Geometry check sheet. Reference: the model listing, model coordinates, mm. A direction names the side the tool comes from. Coordinates: 2 decimals unless noted, no trailing zeros. Write each loop counter-clockwise with the first axis right and the second up, starting at its lowest first coordinate (ties: lowest second). Pieces come first, ordered by that corner, then holes. Notation, with made-up numbers: (8, 51) -> (21, 51) arc R31 cw to (21, 89) -> close; hole circle Ø1 at (77, 7). An arc over 180 degrees is marked (long way). Use a Markdown table: item, result.
```python
from build123d import *

# Parameters (mm, degrees)
F1_DEPTH      = 6.35
F2_W          = 1.3509193668
F2_H          = 10.8486381359
F3_DEPTH      = 2
F5_DEPTH      = 3
F7_R          = 5
F8_T1_DEPTH   = 22.7018387336
F9_T1_DEPTH   = 22.7018387336
F10_T1_DEPTH  = 37.7293119504
F11_T1_DEPTH  = 50.3092406281
F11_T3_DEPTH  = 50.3092406281
F11_T8_DEPTH  = 71.0975509994
F11_T13_DEPTH = 71.0975509994
F12_R         = 1
F13_R         = 1
F14_R         = 1
F15_R         = 1


# Not quite as in the source:
# - a fillet or chamfer that OpenCascade refuses, or shapes differently, is made with other operations: its cross-section is extruded or revolved along the edge and cut away or added


with BuildPart() as f1:
    # F0 (on Top) → F1 (new body)
    with BuildSketch(Plane.XY):
        Polygon((0, -66.0772249103), (0, 35.7286036015), (-4.0004998446, 10.6220170856), (-4.0004998446, -13.1050860509), (-33.7973274291, -28.5552926362), (-33.7973274291, -40.1429459453), (-4.2763971724, -40.1429459453), (-4.2763971724, -50.6270192564), (-13.1050860509, -62.766470015), (-13.1050860509, -69.3879872561), align=None)
    extrude(amount=F1_DEPTH)

    # F2 (on face) → F3 (join)
    with BuildSketch(Plane.XY.offset(6.35)):
        with Locations((-0.6754596834, 8.3060876932)):
            Rectangle(F2_W, F2_H)
    extrude(amount=F3_DEPTH)

    # F4 (on Right) → F5 (join)
    with BuildSketch(Plane.YZ):
        with BuildLine():
            Line((-69.653019309, 0), (-54.4461198151, 0))
            Line((-54.4461198151, 0), (-59.1908343158, 12.4009543867))
            ThreePointArc((-59.1908343158, 12.4009543867), (-61.0264090525, 14.733305135), (-63.8606947699, 15.6142245978))
            Line((-63.8606947699, 15.6142245978), (-66.3944035769, 15.6142245978))
            Line((-66.3944035769, 15.6142245978), (-69.653019309, 0))
        make_face()
    extrude(amount=-F5_DEPTH)

    # F6: F1 across face


with BuildPart() as f1_1:
    add(f1.part)
    add(f1.part.mirror(Plane(origin=(0, -20.6881401181, 4.0270783), x_dir=(0, 1, 0), z_dir=(1, 0, 0))))

    # F7
    f7_edges = [f1_1.edges().sort_by_distance(p)[0] for p in [
        (-18.898914, -20.830189, 6.35),
        (18.898914, -20.830189, 6.35),
    ]]
    fillet(f7_edges, radius=F7_R)

    # F8: fillet of radius 5 on 1 edges, made by hand

    # F8_s2 → F8_t1 (cut)
    with BuildSketch(Plane.YZ.offset(-11.3509193668)):
        with BuildLine():
            ThreePointArc((13.7304067612, 6.35), (11.9664747387, 7.822135955), (9.7304067612, 8.35))
            Line((9.7304067612, 8.35), (13.7304067612, 8.35))
            Line((13.7304067612, 8.35), (13.7304067612, 6.35))
        make_face()
    extrude(amount=F8_T1_DEPTH, mode=Mode.SUBTRACT)

    # F9: fillet of radius 5 on 1 edges, made by hand

    # F9_s2 → F9_t1 (cut)
    with BuildSketch(Plane.YZ.offset(-11.3509193668)):
        with BuildLine():
            ThreePointArc((2.8817686252, 6.35), (4.6457006477, 7.822135955), (6.8817686252, 8.35))
            Line((6.8817686252, 8.35), (2.8817686252, 8.35))
            Line((2.8817686252, 8.35), (2.8817686252, 6.35))
        make_face()
    extrude(amount=F9_T1_DEPTH, mode=Mode.SUBTRACT)

    # F10: fillet of radius 1 on 1 edges, made by hand

    # F10_s2 → F10_t1 (cut)
    with BuildSketch(Plane.XY.offset(-15.6896559752)):
        with BuildLine():
            ThreePointArc((-0.9875420089, 29.5309258493), (0, 30.3735702625), (0.9875420089, 29.5309258493))
            Line((0.9875420089, 29.5309258493), (0, 35.7286036015))
            Line((0, 35.7286036015), (-0.9875420089, 29.5309258493))
        make_face()
    extrude(amount=F10_T1_DEPTH, mode=Mode.SUBTRACT)

    # F11: chamfer of 8 x 1.4106158457 on 2 edges, made by hand

    # F11_s2 → F11_t1 (cut)
    with BuildSketch(Plane.YZ.offset(-54.5856378004)):
        Polygon((-32.1429459453, 6.35), (-40.1429459453, 4.9393841543), (-40.1429459453, 6.35), align=None)
    extrude(amount=F11_T1_DEPTH, mode=Mode.SUBTRACT)

    # F11_s4 → F11_t3 (cut)
    with BuildSketch(Plane.YZ.offset(4.2763971724)):
        Polygon((-32.1429459453, 6.35), (-40.1429459453, 4.9393841543), (-40.1429459453, 6.35), align=None)
    extrude(amount=F11_T3_DEPTH, mode=Mode.SUBTRACT)


with BuildPart() as f11_tool6:
    # F11_s7 → F11_t8 (new body)
    with BuildSketch(Plane.YZ.offset(-54.5856378004)):
        Polygon((-32.1429459453, 6.35), (-40.1429459453, 4.9393841543), (-40.1429459453, 6.35), align=None)
    extrude(amount=F11_T8_DEPTH)

    split(bisect_by=Plane.YZ.offset(4.2763971724), keep=Keep.TOP)


with BuildPart() as f1_2:
    add(f1_1.part)

    # F11_t5: cut F11_tool6
    add(f11_tool6.part, mode=Mode.SUBTRACT)


with BuildPart() as f11_tool11:
    # F11_s12 → F11_t13 (new body)
    with BuildSketch(Plane.YZ.offset(54.5856378004)):
        Polygon((-32.1429459453, 6.35), (-40.1429459453, 4.9393841543), (-40.1429459453, 6.35), align=None)
    extrude(amount=-F11_T13_DEPTH)

    split(bisect_by=Plane.YZ.offset(-4.2763971724), keep=Keep.BOTTOM)


with BuildPart() as f1_3:
    add(f1_2.part)

    # F11_t10: cut F11_tool11
    add(f11_tool11.part, mode=Mode.SUBTRACT)

    # F12
    f12_edges = [f1_3.edges().sort_by_distance(p)[0] for p in [
        (-3, -58.03326, 9.375477),
    ]]
    fillet(f12_edges, radius=F12_R)

    # F13
    f13_edges = [f1_3.edges().sort_by_distance(p)[0] for p in [
        (3, -58.03326, 9.375477),
    ]]
    fillet(f13_edges, radius=F13_R)

    # F14
    f14_edges = [f1_3.edges().sort_by_distance(p)[0] for p in [
        (4.0005, -4.057628, 6.35),
        (-4.0005, -4.057628, 6.35),
        (-4.276397, -41.384983, 6.35),
        (4.276397, -41.384983, 6.35),
    ]]
    fillet(f14_edges, radius=F14_R)

    # F15
    f15_edges = [f1_3.edges().sort_by_distance(p)[0] for p in [
        (4.0005, -1.241534, 0),
        (-4.0005, -1.241534, 0),
        (4.276397, -45.384983, 0),
    ]]
    fillet(f15_edges, radius=F15_R)


solid = f1_3.part
```
Item 1: Thickness scan on L1, parallel to Y at x = -9, z = 4.5; L2, parallel to Z at x = -14, y = -40; L3, parallel to X at y = -6.5, z = 4.5. Record the ranges inside material, lowest first. Write a range as [from, to].
Answer block:
| item | result |
|---|---|
| L1 | y = [-68.35, -57.12], [-40.14, -16.96] |
| L2 | z = [0, 4.96] |
| L3 | x = [-4, 4] |
Item 2: Section check A-A on z = 3.5. Record the boundary of the cut face in (x, y).
Answer block:
| item | result |
|---|---|
| outline | (-33.8, -40.14) -> (-4.28, -40.14) -> (-4.28, -50.63) -> (-13.11, -62.77) -> (-13.11, -69.39) -> (-3, -66.84) -> (-3, -68.92) -> (3, -68.92) -> (3, -66.84) -> (13.11, -69.39) -> (13.11, -62.77) -> (4.28, -50.63) -> (4.28, -40.14) -> (33.8, -40.14) -> (33.8, -29.1) -> (4, -13.65) -> (4, 10.62) -> (0.99, 29.53) arc R1 ccw to (-0.99, 29.53) -> (-4, 10.62) -> (-4, -13.65) -> (-33.8, -29.1) -> close |
Item 3: Section check B-B on y = -43. Record the boundary of the cut face in (x, z), then the cut area to 3 significant figures.
Answer block:
| item | result |
|---|---|
| outline | (-4.28, 0) -> (3.28, 0) arc R1 ccw to (4.28, 1) -> (4.28, 5.35) arc R1 ccw to (3.28, 6.35) -> (-3.28, 6.35) arc R1 ccw to (-4.28, 5.35) -> close |
| area | 53.7 mm^2 |
Item 4: Section check C-C on y = 18. Record the boundary of the cut face in (x, z).
Answer block:
| item | result |
|---|---|
| outline | (-2.82, 0) -> (2.82, 0) -> (2.82, 6.35) -> (-2.82, 6.35) -> close |
Item 5: Depth check by flat-ended pin: P1, Ø3, axis at x = -17, y = -42.5, coming from the +Z side; P2, Ø4, axis at x = -15, z = 1.5, coming from the -Y side; P3, Ø8, axis at x = -19.5, z = 4.5, coming from the -Y side; P4, Ø3.5, axis at y = -1.5, z = 2.5, coming from the -X side. Enter the tip coordinate at first touch or a pass-through.
Answer block:
| item | result |
|---|---|
| P1 | passes through |
| P2 | stops at y = -69.39 |
| P3 | stops at y = -40.14 |
| P4 | stops at x = -4 |
Item 6: Tool access check on faces 1 (the flat face through (-0.028, -58.017, 9.333)), 2 (the flat face through (-1.351, 8, 7)), 3 (the flat face through (3, -64, 9)). Record the directions out of +Z, -Z, +X, -X, +Y, -Y that give a thin tool (end or side, any length) a straight path to the whole face; none if there is none.
Answer block:
| item | result |
|---|---|
| face 1 | +Z, +X, -X |
| face 2 | +Z, -X, +Y |
| face 3 | +Z, -Y |
Item 7: Mould release check, pull along Y, two halves, no side actions. Record for faces 4 (the flat face through (-18.751, -36.087, 5.655)), 5 (the flat face through (-33.797, -34, 2)), 6 (the cylindrical face through (-0.02, 30.373, 3.131)): +Y half, -Y half, draft (parallel to the pull), parting line (faces both ways), or undercut.
Answer block:
| item | result |
|---|---|
| face 4 | undercut |
| face 5 | draft |
| face 6 | +Y half |
